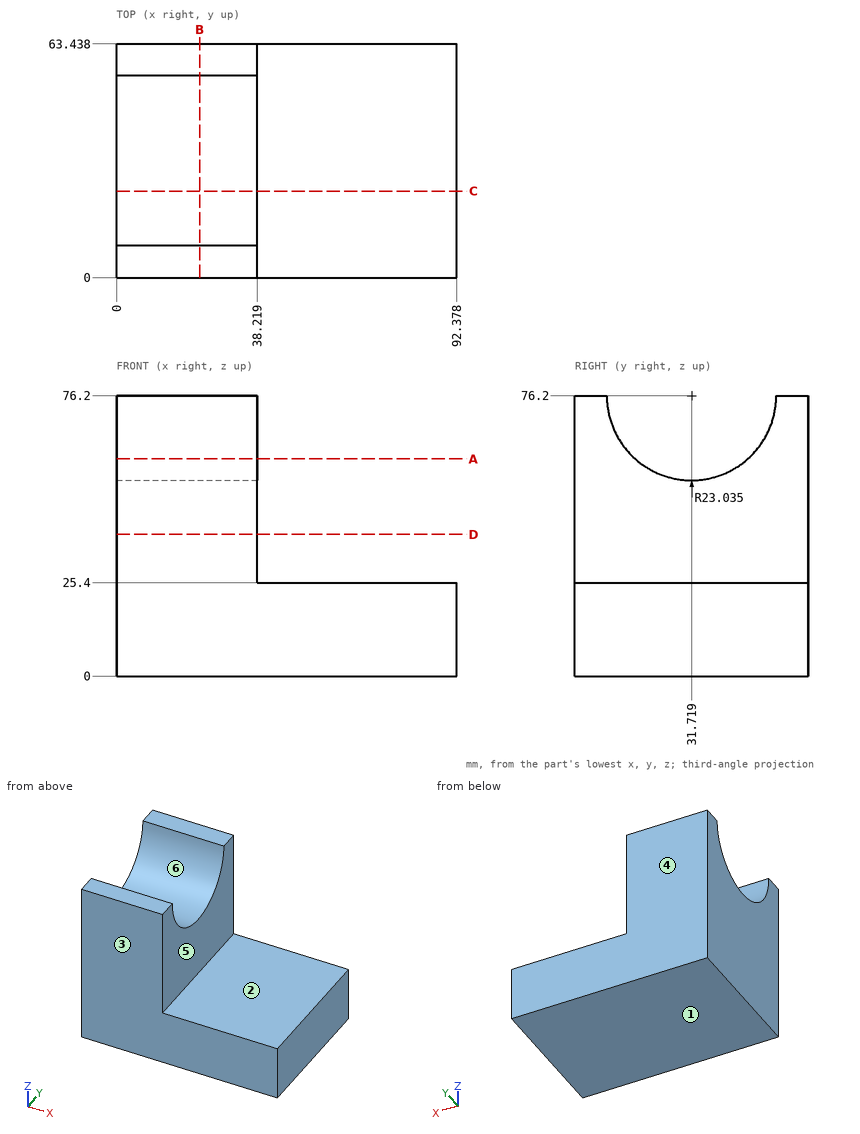
Here's the drawing with two shaded views (mm, measured from the low corner). I have some questions. A direction names the side the tool comes from. Coordinates: 2 decimals unless noted, no trailing zeros. Order: outer loops, then holes, each group sorted by start corner. A loop starts at its lowest first (then second) coordinate and runs counter-clockwise, first axis right, second up. Notation, with made-up numbers: M 89,4 L 138,4 A15 ccw 138,15 Z; hole C 53.5,57.5 d11. An arc over 180 degrees is marked long. Answer as CSV lines item,"result".
Item 1: Imagine slicing it at D-D on z = 38.5. Write out the boundary of the cut face in (x, y).
Results found:
outline,"M 0,0 L 38.22,0 L 38.22,63.44 L 0,63.44 Z"
Item 2: Imagine slicing it at A-A on z = 59. Write out the boundary of the cut face in (x, y).
Results found:
outline,"M 0,0 L 38.22,0 L 38.22,16.4 L 0,16.4 Z; M 0,47.04 L 38.22,47.04 L 38.22,63.44 L 0,63.44 Z"
Item 3: If I drill on line 1 (X direction, y = 54, z = 48); line 2 (Z direction, x = 50.5, y = 55.5); line 3 (Z direction, x = 35, y = 51) (1 decimal), over which ranges is the centre line in solid material (lowest first)?
Results found:
line 1,"0 to 38.22"
line 2,"0 to 25.4"
line 3,"0 to 63.6"
Item 4: Imagine slicing it at C-C on y = 23.5. Write out the boundary of the cut face in (x, z).
Results found:
outline,"M 0,0 L 92.38,0 L 92.38,25.4 L 38.22,25.4 L 38.22,54.68 L 0,54.68 Z"
Item 5: On a 3-axis mill with a long thin cutter (end or side, diameter ignored), from which of +Z, -Z, +X, -X, +Y, -Y can I reach the whole of each face in a straight line? I mean the marked faces 1 and 2. Say none if no direction works.
Results found:
face 1,"-Z, +X, -X, +Y, -Y"
face 2,"+Z, +X, +Y, -Y"
Item 6: We'd pull the mould along Y, two halves only. Please class the marked faces 3, 4, 5 and 6: +Y half, -Y half, draft (parallel to the pull), parting line (faces both ways), or undercut.
Results found:
face 3,"-Y half"
face 4,"+Y half"
face 5,"draft"
face 6,"undercut"
Item 7: For pin 1 (8 mm diameter, centred on x = 46.5, z = 31.5, fed in from -Y); pin 2 (12 mm diameter, centred on x = 78.5, y = 24, fed in from +Z); pin 3 (1.5 mm diameter, centred on y = 54, z = 51.5, fed in from +X), each with a flat end and sliding along its axis, tell me the tip position at first contact or that it passes through.
Results found:
pin 1,"through"
pin 2,"z = 25.4"
pin 3,"x = 38.22"
Item 8: Imagine slicing it at B-B on x = 22.5. Write out the boundary of the cut face in (y, z) (1 decimal).
Results found:
outline,"M 0,0 L 63.4,0 L 63.4,76.2 L 54.8,76.2 A23 cw 8.7,76.2 L 0,76.2 Z"
